Source: three-view drawing plus pictorial views. Frame: mm from the lowest corner of the part. A direction names the side the tool comes from. Give positions to 0.01 mm unless a question says otherwise; leave off trailing zeros. Order: outer loops, then holes, each group sorted by start corner. A loop starts at its lowest first (then second) coordinate and runs counter-clockwise, first axis right, second up. Notation, with made-up numbers: M 62,72 L 73,72 A27 cw 73,93 Z; hole C 49,8 d4. An arc over 180 degrees is marked long. Use CSV: the item, a comma, the result in double quotes. Start each with the question number.
Item 1: First-contact query: pin 1 (6 mm diameter, centred on x = 13.5, z = 16, fed in from +Y); pin 2 (5 mm diameter, centred on y = 7.5, z = 15.5, fed in from +X). Flat tips, straight axial feed; report the tip coordinate or a pass-through.
Item 2: Access query for the marked faces 1 and 2. Directions: +Z, -Z, +X, -X, +Y, -Y. A direction counts if a zero-diameter tool reaches every point of the face in a straight line with its end or side. Return the directions, or none.
Item 3: Section query A-A on z = 7.25. Return loops of the section in (x, y), and give its area (3 significant figures).
Item 4: Ray query, probe 1 along X at (y, z) = (1.5, 9); probe 2 along Y at (x, z) = (14.5, 3). Return the intervals inside material, ascending. Write a range as from..to.
Item 5: Section query C-C on x = 17. Return loops of the section in (y, z), and give its area (3 significant figures).
Item 6: Section query B-B on y = 3.5. Return loops of the section in (x, z).
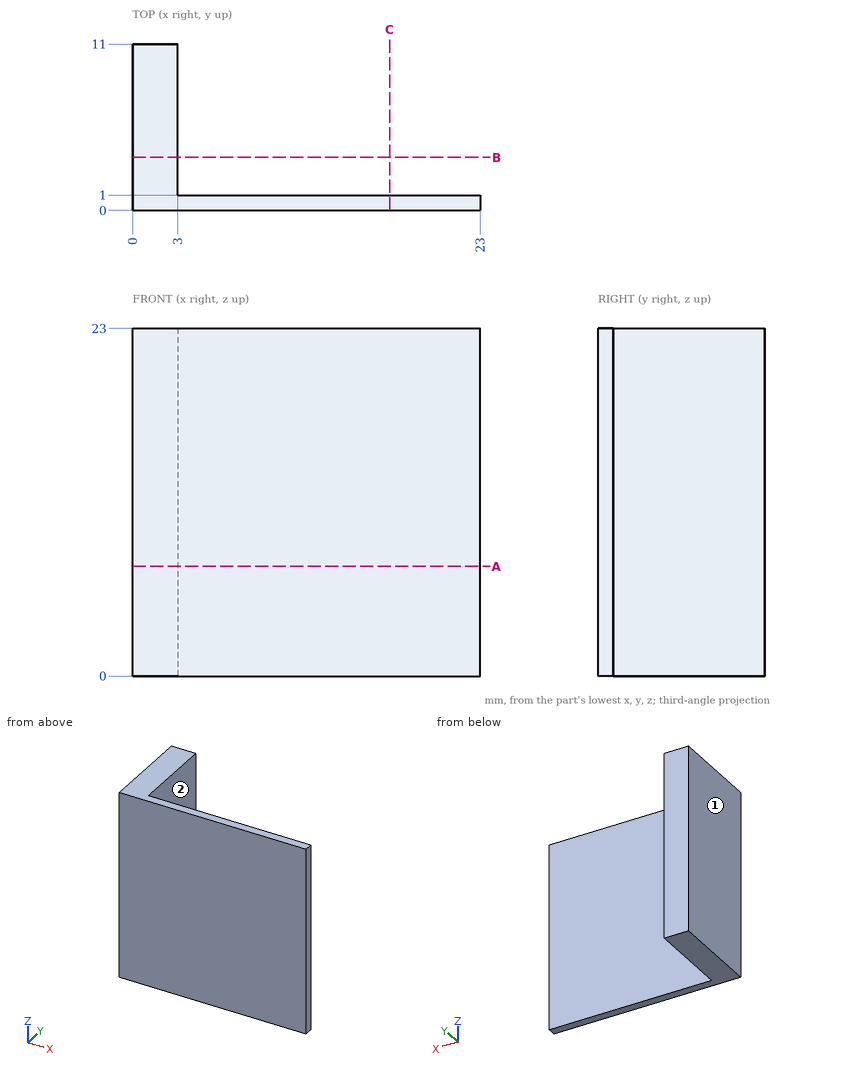
Verdict:
1,pin 1,"y = 1"
1,pin 2,"x = 3"
2,face 1,"+Z, -Z, -X, +Y, -Y"
2,face 2,"+Z, -Z, +X, +Y"
3,outline,"M 0,0 L 23,0 L 23,1 L 3,1 L 3,11 L 0,11 Z"
3,area,"53.0 mm2"
4,probe 1,"0..3"
4,probe 2,"0..1"
5,outline,"M 0,0 L 1,0 L 1,23 L 0,23 Z"
5,area,"23.0 mm2"
6,outline,"M 0,0 L 3,0 L 3,23 L 0,23 Z"
